CAD build for the part. Positions are in the model's coordinates, mm. A direction names the side the tool comes from. Give positions to 0.01 mm unless a question says otherwise; leave off trailing zeros. Order: outer loops, then holes, each group sorted by start corner. A loop starts at its lowest first (then second) coordinate and runs counter-clockwise, first axis right, second up. Notation, with made-up numbers: (67, 19.5) -> (122, 19.5) arc R20 cw to (122, 27.5) -> close; hole circle Ø8 at (0, 55). An arc over 180 degrees is marked (long way). Answer as CSV lines item,"result".
```python
from build123d import *

# Parameters (mm, degrees)
SKETCH_2_R          = 12
SKETCH_2_R_2        = 1.5
EXTRUDE_1_DEPTH     = 2
SKETCH_3_R          = 3.5
EXTRUDE_2_DEPTH     = 15
CUT_EXTRUDE_1_DEPTH = 22.377558326


with BuildPart() as part:
    # 草图2 → 凸台-拉伸1 (new body)
    with BuildSketch(Plane(origin=(0, 0, 0), x_dir=(1, 0, 0), z_dir=(0, 1, 0))):
        with Locations(Location((0, 0, 0), (0, 0, 270))):
            Circle(SKETCH_2_R)
        with Locations(Location((0, 7, 0), (0, 0, 270))):
            Circle(SKETCH_2_R_2, mode=Mode.SUBTRACT)
        with Locations(Location((7, 0, 0), (0, 0, 270))):
            Circle(SKETCH_2_R_2, mode=Mode.SUBTRACT)
        with Locations(Location((0, -7, 0), (0, 0, 270))):
            Circle(SKETCH_2_R_2, mode=Mode.SUBTRACT)
        with Locations(Location((-7, 0, 0), (0, 0, 270))):
            Circle(SKETCH_2_R_2, mode=Mode.SUBTRACT)
    extrude(amount=EXTRUDE_1_DEPTH)

    # 草图3 → 凸台-拉伸2 (add)
    with BuildSketch(Plane.XZ):
        with Locations(Location((0, 0, 0), (0, 0, 270))):
            Circle(SKETCH_3_R)
        with BuildLine():
            Line((-1.661324773, 2), (1.661324773, 2))
            ThreePointArc((1.661324773, 2), (0, -2.6), (-1.661324773, 2))
        make_face(mode=Mode.SUBTRACT)
    extrude(amount=-EXTRUDE_2_DEPTH)

    # 草图4 → 切除-拉伸1 (cut, through all)
    with BuildSketch(Plane(origin=(0, 2, 0), x_dir=(1, 0, 0), z_dir=(0, 1, 0))):
        with BuildLine():
            Line((-1.661324773, -2), (1.661324773, -2))
            ThreePointArc((1.661324773, -2), (0, 2.6), (-1.661324773, -2))
        make_face()
    extrude(amount=-CUT_EXTRUDE_1_DEPTH, mode=Mode.SUBTRACT)


solid = part.part
```
1) Which spindle directions (+Z, -Z, +X, -X, +Y, -Y) get a long thin tool onto all of the face, cutting with end or side? Do faces 4 (the flat face through (0, 8, 2)), 5 (the flat face through (0, 15, 2.4)), 6 (the flat face through (2.8, 2, 2.5)). Say none if no direction does.
Data:
face 4,"+Y, -Y"
face 5,"+Z, -Z, +X, -X, +Y"
face 6,"+Y"
2) Wall check: line 1 along X through (y, z) = (0.6, 0); line 2 along X through (y, z) = (13.5, 0); line 3 along Y through (x, z) = (10.5, -3.5). Give the ranges that are in metal, low to high. Write a range as [from, to].
Data:
line 1,"x = [-12, -8.5], [-5.5, -2.6], [2.6, 5.5], [8.5, 12]"
line 2,"x = [-3.5, -2.6], [2.6, 3.5]"
line 3,"y = [0, 2]"
3) Band-saw the part on A-A, the plane z = 0. Write the cut outline in (x, y).
Data:
outline,"(-12, 0) -> (-8.5, 0) -> (-8.5, 2) -> (-12, 2) -> close; (-5.5, 0) -> (-2.6, 0) -> (-2.6, 15) -> (-3.5, 15) -> (-3.5, 2) -> (-5.5, 2) -> close; (2.6, 0) -> (5.5, 0) -> (5.5, 2) -> (3.5, 2) -> (3.5, 15) -> (2.6, 15) -> close; (8.5, 0) -> (12, 0) -> (12, 2) -> (8.5, 2) -> close"
4) Band-saw the part on C-C, the plane x = 3. Write the cut outline in (y, z), then the cut area to 3 significant figures.
Data:
outline,"(0, -11.62) -> (2, -11.62) -> (2, -1.8) -> (15, -1.8) -> (15, 1.8) -> (2, 1.8) -> (2, 11.62) -> (0, 11.62) -> close"
area,"93.3 mm2"
5) Band-saw the part on B-B, the plane z = -8. Write the cut outline in (x, y).
Data:
outline,"(-8.94, 0) -> (-1.12, 0) -> (-1.12, 2) -> (-8.94, 2) -> close; (1.12, 0) -> (8.94, 0) -> (8.94, 2) -> (1.12, 2) -> close"
6) Pin check, flat tips, straight feed: P1, Ø1.5, axis at y = 3.5, z = 6.5, coming from the +X side; P2, Ø2, axis at y = 10, z = -1, coming from the -X side; P3, Ø8, axis at y = 11, z = 1, coming from the +X side; P4, Ø5, axis at x = 0, z = 7, coming from the +Y side. Stop position of each tip, or through.
Data:
P1,"passes through"
P2,"stops at x = -3.5"
P3,"stops at x = 3.5"
P4,"stops at y = 2"
7) Pull direction Z, two halves, no side cores. Call faces 1 (the cylindrical face through (-8.464, 0.986, -0.325)), 2 (the cylindrical face through (-3.417, 8.409, 0.759)), 3 (the flat face through (3, 0, 0)): pulls with the +Z half, pulls with the -Z half, needs draft (parallel to the pull), parting line crosses it, or undercut.
Data:
face 1,"undercut"
face 2,"parting line crosses it"
face 3,"needs draft"
8) Band-saw the part on D-D, the plane x = 7. Write the cut outline in (y, z), then the cut area to 3 significant figures.
Data:
outline,"(0, -9.75) -> (2, -9.75) -> (2, -1.5) -> (0, -1.5) -> close; (0, 1.5) -> (2, 1.5) -> (2, 9.75) -> (0, 9.75) -> close"
area,"33.0 mm2"
